Part model, mm, in its own coordinate system. Give positions to 0.01 mm unless a question says otherwise; leave off trailing zeros. Write each loop counter-clockwise with the first axis right and the second up, starting at its lowest first coordinate (ties: lowest second). Pieces come first, ordered by that corner, then holes.
Autodesk Inventor part; units mm, degrees
ref_plane "YZ Plane" through (0, 0, 0) normal (1, 0, 0) x (0, 1, 0)
ref_plane "XZ Plane" through (0, 0, 0) normal (0, 1, 0) x (-1, 0, 0)
ref_plane "XY Plane" through (0, 0, 0) normal (0, 0, 1) x (1, 0, 0)
sketch "Sketch1" plane through (0, 0, 0) normal (0, 1, 0) x (-1, 0, 0)
  line L0 (0, 18.5) -> (0, 18.5)
  line L1 (-9, 9.5) -> (-9, -9.5)
  line L2 (0, -18.5) -> (0, -18.5)
  line L3 (9, -9.5) -> (9, 9.5)
  arc A0 (9, 9.5) -> (0, 18.5) centre (0, 9.5) ccw
  arc A1 (0, -18.5) -> (9, -9.5) centre (0, -9.5) ccw
  arc A2 (-9, -9.5) -> (0, -18.5) centre (0, -9.5) ccw
  arc A3 (0, 18.5) -> (-9, 9.5) centre (0, 9.5) ccw
  point P0 (0, 0)
  point P1 (-9, -18.5)
  point P2 (-9, 18.5)
  point P3 (9, -18.5)
  point P4 (0, -18.5)
  dimension "d0" = 18
  dimension "d1" = 37
  dimension "d2" = 18.5
  dimension "d3" = 9
  dimension "d4" = 9
extrude "Extrusion1" add sketch "Sketch1" along normal blind 69
sketch "Sketch2" plane through (0, 69, 0) normal (0, 1, 0) x (1, 0, 0)
  line L0 (9, -9.5) -> (9, 9.5)
  line L1 (9, 2) -> (7, 2)
  line L2 (7, 2) -> (7, -2)
  line L3 (7, -2) -> (9, -2)
  line L4 (9, -2) -> (9, 2)
  point P0 (0, 0)
  dimension "d7" = 2
  dimension "d8" = 4
  dimension "d9" = 2
extrude "Extrusion2" add sketch "Sketch2" along normal blind 1
equation "\"d8\" = 2 * d7"
properties part number "Battery"
1) Saw through at A-A, the plane z = 12. Write the cut outline in (x, y), then the cut area to 3 significant figures.
Answers follow:
outline: (-8.65, 0) - (8.65, 0) - (8.65, 69) - (-8.65, 69) - close
area: 1,190 mm2
2) Pin check, flat tips, straight feed: pin 1 Ø4 at (x, y) = (2.5, 22.5) entering from +Z; pin 2 Ø0.5 at (x, y) = (7.5, 69.5) entering from +Z; pin 3 Ø1.5 at (x, z) = (-2.5, 4) entering from +Y. Stop position of each tip, or through.
Answers follow:
pin 1: stops at z = 18.49
pin 2: stops at z = 2
pin 3: stops at y = 69
3) Saw through at B-B, the plane y = 52. Write the cut outline in (x, z).
Answers follow:
outline: (-9, -9.5) arc R9 ccw to (9, -9.5) - (9, 9.5) arc R9 ccw to (-9, 9.5) - close
4) Wall check: L1, parallel to Y at x = -1.75, z = -5; L2, parallel to Z at x = -0.5, y = 62; L3, parallel to Z at x = 5.5, y = 56. Give the ranges that are in metal, low to high.
Answers follow:
L1: y = 0 to 69
L2: z = -18.49 to 18.49
L3: z = -16.62 to 16.62
